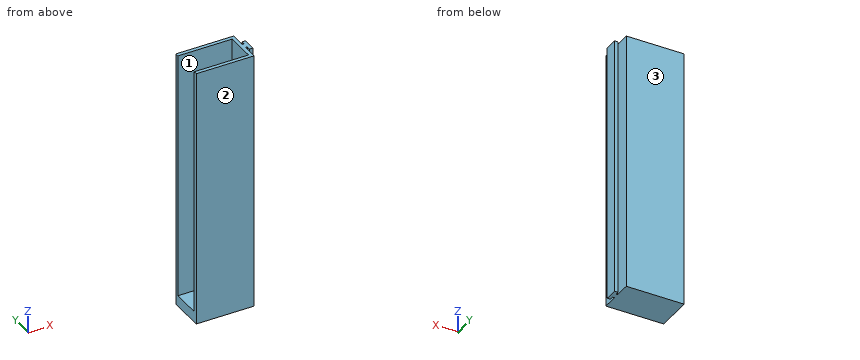
```python
from build123d import *

# Parameters (mm, degrees)
SKETCH_W     = 40
SKETCH_H     = 25
PAD_DEPTH    = 180
SKETCH001_W  = 39.599754
SKETCH001_H  = 20
POCKET_DEPTH = 172.5
SKETCH002_W  = 1.967115
SKETCH002_H  = 3.9
PAD001_DEPTH = 180
SKETCH003_W  = 2.3
SKETCH003_H  = 9
PAD002_DEPTH = 180


with BuildPart() as part:
    # Sketch → Pad (new body)
    with BuildSketch(Plane.XY):
        Rectangle(SKETCH_W, SKETCH_H)
    extrude(amount=PAD_DEPTH)

    # Sketch001 (on Face6 of Pad) → Pocket (cut)
    with BuildSketch(Plane.XY.offset(180)):
        with Locations((-2.299877, 0)):
            Rectangle(SKETCH001_W, SKETCH001_H)
    extrude(amount=-POCKET_DEPTH, mode=Mode.SUBTRACT)

    # Sketch002 (on Face5 of Pocket) → Pad001 (join)
    with BuildSketch(Plane.XY.offset(180)):
        with Locations((20.2164425, 0)):
            Rectangle(SKETCH002_W, SKETCH002_H)
    extrude(amount=-PAD001_DEPTH)

    # Sketch003 (on DatumPlane) → Pad002 (join)
    with BuildSketch(Plane.XY.offset(180)):
        with Locations((22.35, -0.0960954544)):
            Rectangle(SKETCH003_W, SKETCH003_H)
    extrude(amount=-PAD002_DEPTH)


solid = part.part
```
Can you work these out from the model? Positions are in its coordinate system, mm. Face numbers are marked on the shaded views. Give positions to 0.01 mm unless a question says otherwise; leave off trailing zeros. Write each loop counter-clockwise with the first axis right and the second up, starting at its lowest first coordinate (ties: lowest second). Pieces come first, ordered by that corner, then holes. Notation, with made-up numbers: (38, 77) -> (85, 77) arc R24 ccw to (85, 106) -> close; hole circle Ø1 at (28.5, -33). An arc over 180 degrees is marked (long way). Write item = value, one per line.
(1) I'm going to push flat-ended pins straight in: P1, Ø4, axis at y = -1, z = 34.5, coming from the -X side; P2, Ø10, axis at x = -3.5, y = -4.5, coming from the +Z side; P3, Ø8.5, axis at y = -9, z = 97, coming from the +X side. Where does each tip first touch, or does it pass through?
Worked out:
P1 = 17.5
P2 = 7.5
P3 = 20
(2) Thinking about a two-plate mould opening in Y: for the marked faces 1, 2 and 3, which applies, released by +Y, released by -Y, zero draft, split by the parting line, or undercut?
Worked out:
face_1 = undercut
face_2 = released by -Y
face_3 = released by +Y
(3) Suppose I cut it at C-C on y = -7.5. Write out the boundary of the cut face in (x, z).
Worked out:
outline = (-20, 0) -> (20, 0) -> (20, 180) -> (17.5, 180) -> (17.5, 7.5) -> (-20, 7.5) -> close
(4) Suppose I cut it at D-D on y = -0.25. Write out the boundary of the cut face in (x, z).
Worked out:
outline = (-20, 0) -> (23.5, 0) -> (23.5, 180) -> (17.5, 180) -> (17.5, 7.5) -> (-20, 7.5) -> close
(5) Suppose I cut it at A-A on x = 0. Write out the boundary of the cut face in (y, z), then the cut area to 3 significant figures.
Worked out:
outline = (-12.5, 0) -> (12.5, 0) -> (12.5, 180) -> (10, 180) -> (10, 7.5) -> (-10, 7.5) -> (-10, 180) -> (-12.5, 180) -> close
area = 1,050 mm^2
(6) Suppose I cut it at B-B on z = 133.5. Write out the boundary of the cut face in (x, y).
Worked out:
outline = (-20, -12.5) -> (20, -12.5) -> (20, -1.95) -> (21.2, -1.95) -> (21.2, -4.6) -> (23.5, -4.6) -> (23.5, 4.4) -> (21.2, 4.4) -> (21.2, 1.95) -> (20, 1.95) -> (20, 12.5) -> (-20, 12.5) -> (-20, 10) -> (17.5, 10) -> (17.5, -10) -> (-20, -10) -> close
(7) I need wall thicknesses on probe 1 along X at (y, z) = (2.5, 11); probe 2 along Y at (x, z) = (-10, 72.5); probe 3 along X at (y, z) = (1.75, 154). Which ranges of each line are inside material? Lowest first, please. Write a range as from..to.
Worked out:
probe_1 = 17.5..20, 21.2..23.5
probe_2 = -12.5..-10, 10..12.5
probe_3 = 17.5..23.5
